Here's how the part is built. I have some questions about the finished solid (model axes, mm). A direction names the side the tool comes from. Coordinates: 2 decimals unless noted, no trailing zeros. Order: outer loops, then holes, each group sorted by start corner. A loop starts at its lowest first (then second) coordinate and runs counter-clockwise, first axis right, second up. Notation, with made-up numbers: M -8,17 L 12,17 A12 cw 12,39 Z; hole C 51.25,58 d2. An arc over 180 degrees is marked long. Answer as CSV lines item,"result". Start each with the question number.
```python
from build123d import *

# Parameters (mm, degrees)
BOSS_EXTRUDE1_DEPTH = 5
SKETCH2_W           = 20
SKETCH2_H           = 20
CUT_EXTRUDE1_DEPTH  = 5
SKETCH5_R           = 1.5
CUT_EXTRUDE2_DEPTH  = 36.707142143
SKETCH6_W           = 16
SKETCH6_H           = 0.8
CUT_EXTRUDE3_DEPTH  = 36.707142143


with BuildPart() as part:
    # Sketch1 → Boss-Extrude1 (new body)
    with BuildSketch(Plane.XY):
        with BuildLine():
            Line((-21.09, 25), (21.09, 25))
            ThreePointArc((21.09, 25), (23.854787514, 23.854787514), (25, 21.09))
            Line((25, 21.09), (25, -21.09))
            ThreePointArc((25, -21.09), (23.854787514, -23.854787514), (21.09, -25))
            Line((21.09, -25), (20.757353845, -25))
            Line((20.757353845, -25), (-21.09, -25))
            ThreePointArc((-21.09, -25), (-23.854787514, -23.854787514), (-25, -21.09))
            Line((-25, -21.09), (-25, 21.09))
            ThreePointArc((-25, 21.09), (-23.854787514, 23.854787514), (-21.09, 25))
        make_face()
    extrude(amount=BOSS_EXTRUDE1_DEPTH)

    # Sketch2 → Cut-Extrude1 (cut)
    with BuildSketch(Plane.XY.offset(5)):
        Rectangle(SKETCH2_W, SKETCH2_H)
    extrude(amount=-CUT_EXTRUDE1_DEPTH, mode=Mode.SUBTRACT)

    # Sketch5 → Cut-Extrude2 (cut, through all)
    with BuildSketch(Plane.XY.offset(5)):
        with Locations((-20, 20)):
            Circle(SKETCH5_R)
        with Locations((18.13054205, 20)):
            Circle(SKETCH5_R)
        with Locations((-20, -20)):
            Circle(SKETCH5_R)
        with Locations((20, -20)):
            Circle(SKETCH5_R)
    extrude(amount=-CUT_EXTRUDE2_DEPTH, mode=Mode.SUBTRACT)

    # Sketch6 → Cut-Extrude3 (cut, through all)
    with BuildSketch(Plane(origin=(0, 0, 0), x_dir=(-1, 0, 0), z_dir=(0, 0, -1))):
        with Locations((0, 24.6)):
            Rectangle(SKETCH6_W, SKETCH6_H)
    extrude(amount=-CUT_EXTRUDE3_DEPTH, mode=Mode.SUBTRACT)


solid = part.part
```
1) Which directions (+Z, -Z, +X, -X, +Y, -Y) give clear straight access to the entire face, cutting with the end or side of a thin tool? Please do faces 1 (the face through (10, 0, 3)), 2 (the face through (23.89, -23.82, 2.46)), 3 (the face through (0, 24.2, 2)).
2) Suppose I cut it at A-A on x = -5. Please give me the cut outline in (y, z), plus the area to 3 significant figures.
3) Will these pins go through, and if not, where does the flat tip stop? pin 1 Ø2.5 at (x, y) = (20, -20) entering from +Z; pin 2 Ø2.5 at (x, z) = (2.5, 2.5) entering from +Y; pin 3 Ø12 at (x, y) = (17.5, -13.5) entering from -Z; pin 4 Ø0.6 at (y, z) = (24.5, 2.5) entering from -X.
4) Suppose I cut it at B-B on y = 20. Please give me the cut outline in (x, z), plus the area to 3 significant figures.
5) Suppose I cut it at D-D on z = 4.15. Please give me the cut outline in (x, y), plus the area to 3 significant figures.
6) I need wall thicknesses on line 1 (Y direction, x = -20, z = 3.2); line 2 (Y direction, x = -8.5, z = 2.55). Which ranges of each line are inside material? Lowest first, please. Write a range as [from, to].
7) Suppose I cut it at C-C on y = 3. Please give me the cut outline in (x, z).
8) If we mould it in two halves opening along Y, with no side actions, what happens to faces 4 (the face through (0, 10, 3)), 5 (the face through (-25, 0, 2)), 6 (the face through (-15, 25, 2))? For each: released by +Y, released by -Y, zero draft, split by the parting line, or undercut.
Output:
1,face 1,"+Z, -Z"
1,face 2,"+Z, -Z, +X, -Y"
1,face 3,"+Z, -Z, +Y"
2,outline,"M -25,0 L -10,0 L -10,5 L -25,5 Z; M 10,0 L 24.2,0 L 24.2,5 L 10,5 Z"
2,area,"146 mm²"
3,pin 1,"through"
3,pin 2,"y = 24.2"
3,pin 3,"z = 0"
3,pin 4,"x = -23.46"
4,outline,"M -25,0 L -21.5,0 L -21.5,5 L -25,5 Z; M -18.5,0 L 16.63,0 L 16.63,5 L -18.5,5 Z; M 19.63,0 L 25,0 L 25,5 L 19.63,5 Z"
4,area,"220 mm²"
5,outline,"M -25,-21.09 A3.91 ccw -21.09,-25 L 21.09,-25 A3.91 ccw 25,-21.09 L 25,21.09 A3.91 ccw 21.09,25 L 8,25 L 8,24.2 L -8,24.2 L -8,25 L -21.09,25 A3.91 ccw -25,21.09 Z; hole C -20,-20 d3; hole C -20,20 d3; hole M -10,-10 L 10,-10 L 10,10 L -10,10 Z; hole C 18.13,20 d3; hole C 20,-20 d3"
5,area,"2,050 mm²"
6,line 1,"[-25, -21.5], [-18.5, 18.5], [21.5, 25]"
6,line 2,"[-25, -10], [10, 25]"
7,outline,"M -25,0 L -10,0 L -10,5 L -25,5 Z; M 10,0 L 25,0 L 25,5 L 10,5 Z"
8,face 4,"undercut"
8,face 5,"zero draft"
8,face 6,"released by +Y"
